Input: part model. Units: mm. Frame: model coordinates. A direction names the side the tool comes from. Give positions to 0.01 mm unless a question says otherwise; leave off trailing zeros. Loops run counter-clockwise (first coordinate to the right, second up) from the corner with the lowest first, then second, coordinate; pieces in that order, holes last.
Autodesk Inventor part; units mm, degrees
ref_plane "YZ Plane" through (0, 0, 0) normal (1, 0, 0) x (0, 1, 0)
ref_plane "XZ Plane" through (0, 0, 0) normal (0, 1, 0) x (-1, 0, 0)
ref_plane "XY Plane" through (0, 0, 0) normal (0, 0, 1) x (1, 0, 0)
sketch "Sketch1" plane through (0, 0, 0) normal (0, 0, 1) x (1, 0, 0)
  circle A0 centre (0, 0) radius 45
  circle A1 centre (0, 0) radius 34.925
  circle A2 centre (0, 0) radius 11.075
  dimension "d0" = 90
  dimension "d1" = 69.85
  dimension "d2" = 22.15
extrude "Extrusion1" add sketch "Sketch1" along normal blind 20 contours A1
extrude "Extrusion2" add sketch "Sketch1" against normal blind 10 contours A0
sketch "Sketch2" plane through (0, 0, 20) normal (0, 0, 1) x (1, 0, 0)
  circle A0 centre (12.4625, 21.5857) radius 4
  circle A1 centre (-24.925, 0) radius 4
  circle A2 centre (12.4625, -21.5857) radius 4
  line L0 (-24.925, 0) -> (12.4625, 21.5857) construction
  line L1 (12.4625, 21.5857) -> (12.4625, -21.5857) construction
  line L2 (12.4625, -21.5857) -> (-24.925, 0) construction
  line L3 (12.4625, 21.5857) -> (17.4625, 30.2459) construction
  circle A3 centre (0, 0) radius 34.925
  line L4 (-24.925, 0) -> (-34.925, 0) construction
  line L5 (12.4625, -21.5857) -> (17.4625, -30.2459) construction
  dimension "d7" = 8
  dimension "d8" = 10
extrude "Extrusion3" cut sketch "Sketch2" against normal blind 15 contours A0 | A1 | A2
sketch "Sketch3" plane through (0, 0, 0) normal (0, 0, -1) x (-1, 0, 0)
  circle A0 centre (0, 0) radius 3.475
  circle A1 centre (0, 0) radius 11.075
  line L0 (0, -3.475) -> (-10.5157, -3.475)
  line L1 (0, -3.475) -> (10.5157, -3.475)
  circle A2 centre (0, 0) radius 11.075
  dimension "d11" = 6.95
extrude "Extrusion4" add sketch "Sketch3" against normal blind 5 contours L0 A1 L1 picked at (8.4294, 0.9033)
extrude "Extrusion5" add sketch "Sketch3" against normal blind 30 contours A0
sketch "Sketch4" plane through (0, 0, 30) normal (0, 0, 1) x (1, 0, 0)
  circle A0 centre (0, 0) radius 2.5
  dimension "d16" = 5
extrude "Extrusion6" cut sketch "Sketch4" against normal blind 1.5
sketch "Sketch5" plane through (0, 0, 0) normal (0, 0, -1) x (-1, 0, 0)
  circle A0 centre (0, 0) radius 14.925
  circle A1 centre (0, 0) radius 34.925
  dimension "d19" = 20
extrude "Extrusion7" add sketch "Sketch5" along normal blind 10
sketch "Sketch6" plane through (0, 0, -10) normal (0, 0, -1) x (-1, 0, 0)
  circle A0 centre (12.4625, 21.5857) radius 4
  circle A1 centre (-24.925, 0) radius 4
  circle A2 centre (12.4625, -21.5857) radius 4
  line L0 (12.4625, 21.5857) -> (12.4625, -21.5857) construction
  line L1 (12.4625, -21.5857) -> (12.4625, -6.5031) construction
  line L2 (12.4625, -21.5857) -> (-24.925, 0) construction
  line L3 (-24.925, 0) -> (12.4625, 21.5857) construction
  circle A3 centre (0, 0) radius 14.925 construction
  line L4 (12.4625, -21.5857) -> (7.4625, -12.9254) construction
  circle A4 centre (0, 0) radius 14.925 construction
  line L5 (-24.925, 0) -> (-14.925, 0) construction
  line L6 (12.4625, 21.5857) -> (7.4625, 12.9254) construction
  dimension "d22" = 8
  dimension "d23" = 10
extrude "Extrusion8" cut sketch "Sketch6" against normal blind 10
properties part number "Tractor_Static"
(1) Cut plane B-B (y = 33.5). Return the cut outline in (x, z).
Values follow:
outline: (-30.05, -10) - (30.05, -10) - (30.05, 0) - (9.87, 0) - (9.87, 20) - (-9.87, 20) - (-9.87, 0) - (-30.05, 0) - close
(2) Ray query, probe 1 along Z at (x, y) = (-38, 19.5); probe 2 along Y at (x, z) = (6.5, -4.5); probe 3 along Y at (x, z) = (14.5, 18.5). Return the intervals inside material, ascending.
Values follow:
probe 1: z = -10 to 0
probe 2: y = -44.53 to -13.44, 13.44 to 44.53
probe 3: y = -31.77 to -25.03, -18.14 to 18.14, 25.03 to 31.77
(3) Reachability of faces 1 (the cylindrical face through (0.753, -3.392, 17.325)), 2 (the flat face through (11, 11, -10)), 3 (the flat face through (0, 0, 0)), 4 (the flat face through (0, -3.475, 2)) from +Z, -Z, +X, -X, +Y, -Y: full face, straight path, thin tool, end or side. Return the list, or none.
Values follow:
face 1: +Z
face 2: -Z, +X, -X, +Y, -Y
face 3: -Z
face 4: +Z, -Z
(4) Cut plane C-C (z = 25). Return the cut outline in (x, y) (3 decimals), and give its area (3 significant figures).
Values follow:
outline: circle Ø6.95 at (0, 0)
area: 37.9 mm2
(5) Pin query (flat end, axial travel): pin 1 Ø8 at (x, y) = (-21.5, -20) entering from +Z; pin 2 Ø2.5 at (x, y) = (-12, 21) entering from -Z; pin 3 Ø2.5 at (x, y) = (-26, 0) entering from +Z. Return the tip coordinate at first contact, or that it passes through.
Values follow:
pin 1: stops at z = 20
pin 2: stops at z = 0
pin 3: stops at z = 5
(6) Mould query, pull axis Y, two halves, no side actions, for faces 5 (the flat face through (-8, 8, 20)), 6 (the flat face through (25, 0, 0)), 7 (the cylindrical face through (20.765, -39.923, -4.93)). Classes: +Y half, -Y half, draft (parallel to the pull), parting line (faces both ways), or undercut.
Values follow:
face 5: draft
face 6: undercut
face 7: parting line
(7) Cut plane D-D (y = 9). Return the cut outline in (x, z).
Values follow:
outline: (-44.09, -10) - (-11.91, -10) - (-11.91, 0) - (11.91, 0) - (11.91, -10) - (44.09, -10) - (44.09, 0) - (33.75, 0) - (33.75, 20) - (6.45, 20) - (6.45, 5) - (-6.45, 5) - (-6.45, 20) - (-33.75, 20) - (-33.75, 0) - (-44.09, 0) - close
(8) Cut plane A-A (y = -7). Return the cut outline in (x, z), and give its area (3 significant figures).
Values follow:
outline: (-44.45, -10) - (-13.18, -10) - (-13.18, 0) - (-8.58, 0) - (-8.58, 20) - (-34.22, 20) - (-34.22, 0) - (-44.45, 0) - close; (8.58, 0) - (13.18, 0) - (13.18, -10) - (44.45, -10) - (44.45, 0) - (34.22, 0) - (34.22, 20) - (8.58, 20) - close
area: 1,650 mm2
